Here's the drawing with two shaded views (mm, measured from the low corner). I have some questions. A direction names the side the tool comes from. Round coordinates to 2 decimals unless told otherwise and drop trailing zeros. Loops run counter-clockwise (first coordinate to the right, second up) from the corner with the lowest first, then second, coordinate; pieces in that order, holes last. Notation, with made-up numbers: M 61,-32.75 L 70,-32.75 A22 cw 70,-26.75 Z; hole C -27.5,-33 d3. An arc over 180 degrees is marked long. Answer as CSV lines item,"result".
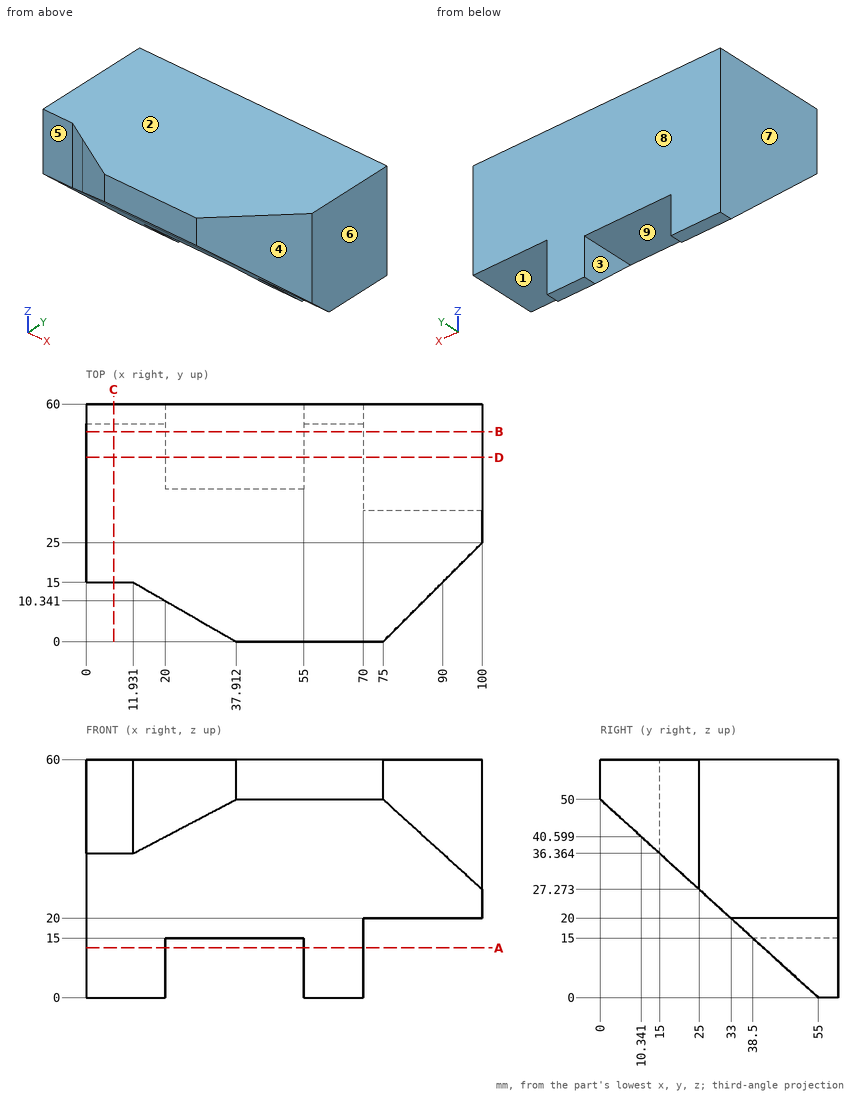
1. I want a section at D-D, the plane y = 46.5. Please give me the cut outline in (x, z).
Evaluation:
outline,"M 0,7.73 L 20,7.73 L 20,15 L 55,15 L 55,7.73 L 70,7.73 L 70,20 L 100,20 L 100,60 L 0,60 Z"
2. Which directions (+Z, -Z, +X, -X, +Y, -Y) give clear straight access to the entire face, cutting with the end or side of a thin tool? Please do the marked faces 1, 2, 3, 4 and 5.
Evaluation:
face 1,"-Z, +X, +Y, -Y"
face 2,"+Z, +X, -X, +Y, -Y"
face 3,"-Z, +Y, -Y"
face 4,"+Z, -Z, +X, -Y"
face 5,"+Z, -Z, -X, -Y"
3. I want a section at A-A, the plane z = 12.5. Please give me the cut outline in (x, y).
Evaluation:
outline,"M 0,41.25 L 20,41.25 L 20,60 L 0,60 Z; M 55,41.25 L 70,41.25 L 70,60 L 55,60 Z"
4. I want a section at C-C, the plane x = 7. Please give me the cut outline in (y, z).
Evaluation:
outline,"M 15,36.36 L 55,0 L 60,0 L 60,60 L 15,60 Z"
5. For P1, Ø16, axis at y = 43.5, z = 10.5, coming from the +X side; P2, Ø1.5, axis at x = 11, y = 26, coming from the -Z side; P3, Ø17, axis at x = 30, y = 48, coming from the -Z side, each with a flat end and sliding along its axis, tell me the tip position at first contact or that it passes through.
Evaluation:
P1,"stops at x = 70"
P2,"stops at z = 25.68"
P3,"stops at z = 15"
6. If I drill on line 1 (Z direction, x = 75.5, y = 25); line 2 (Z direction, x = 92, y = 52); line 3 (X direction, y = 37, z = 16.5), over which ranges is the centre line in solid material (lowest first)? Write a range as [from, to].
Evaluation:
line 1,"z = [27.27, 60]"
line 2,"z = [20, 60]"
line 3,"x = [0, 70]"
7. We'd pull the mould along X, two halves only. Please class the marked faces 6, 7, 8 and 9: pulls with the +X half, pulls with the -X half, needs draft (parallel to the pull), parting line crosses it, or undercut.
Evaluation:
face 6,"pulls with the +X half"
face 7,"pulls with the -X half"
face 8,"needs draft"
face 9,"undercut"
8. I want a section at B-B, the plane y = 53. Please give me the cut outline in (x, z), and give its area (3 significant figures).
Evaluation:
outline,"M 0,1.82 L 20,1.82 L 20,15 L 55,15 L 55,1.82 L 70,1.82 L 70,20 L 100,20 L 100,60 L 0,60 Z"
area,"4,810 mm²"
